Design review of the part built by this model. Coordinates are the model's own, in mm. Face numbers are marked on the shaded views. A direction names the side the tool comes from. Give positions to 0.01 mm unless a question says otherwise; leave off trailing zeros. Write each loop counter-clockwise with the first axis right and the second up, starting at its lowest first coordinate (ties: lowest second). Pieces come first, ordered by that corner, then holes.
```python
from build123d import *

# Parameters (mm, degrees)
F0_R     = 31
F1_DEPTH = 49
F2_R     = 17.5
F4_DEPTH = 52
F6_D     = 3


# Not quite as in the source:
# - the program builds the solid bodies; features that only make, move or delete a surface that nothing else refers to are left out


with BuildPart() as f1:
    # F0 (on Top) → F1 (new body)
    with BuildSketch(Plane.XY):
        Circle(F0_R)
    extrude(amount=F1_DEPTH)

    # F2 (on Top) → F4 (join)
    with BuildSketch(Plane.XY):
        Circle(F2_R)
    extrude(amount=F4_DEPTH)

    # F6 (through all)
    with Locations(Plane.XY.offset(52)):
        with Locations((0, 15), (-15, 0), (0, -15), (15, 0)):
            Hole(F6_D / 2)


solid = f1.part
```
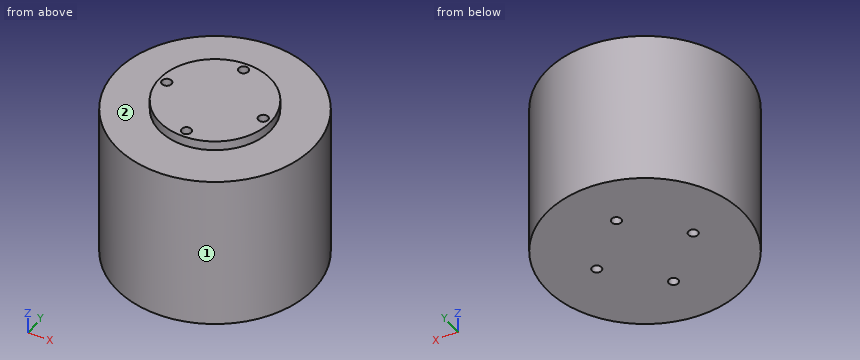
(1) Consider section D-D, the plane y = -15. Give the boundary of the cut face in (x, z).
Resolved:
outline: (-27.13, 0) - (-1.5, 0) - (-1.5, 52) - (-9.01, 52) - (-9.01, 49) - (-27.13, 49) - close; (1.5, 0) - (27.13, 0) - (27.13, 49) - (9.01, 49) - (9.01, 52) - (1.5, 52) - close
(2) Consider section A-A, the plane z = 40. Give the boundary of the cut face in (x, y), then the cut area to 3 significant figures.
Resolved:
outline: circle Ø62 at (0, 0); hole circle Ø3 at (-15, 0); hole circle Ø3 at (0, -15); hole circle Ø3 at (0, 15); hole circle Ø3 at (15, 0)
area: 2,990 mm2
(3) Clearance check with flat-ended pins moving along their axes: P1, Ø8, axis at x = 17, y = 20, coming from the +Z side; P2, Ø2, axis at y = 14.5, z = 14, coming from the -X side; P3, Ø3, axis at x = -5.5, z = 44, coming from the -Y side. State where each tip first meets the part, or that it passes through.
Resolved:
P1: stops at z = 49
P2: stops at x = -27.91
P3: stops at y = -30.74
(4) To check wall thickness, follow L1, parallel to Y at x = 0, z = 30; L2, parallel to Y at x = 1, z = 34. State the ranges of each line that lie inside material, in increasing order.
Resolved:
L1: y = -31 to -16.5, -13.5 to 13.5, 16.5 to 31
L2: y = -30.98 to -16.12, -13.88 to 13.88, 16.12 to 30.98
(5) Consider section B-B, the plane y = 0. Give the boundary of the cut face in (x, z).
Resolved:
outline: (-31, 0) - (-16.5, 0) - (-16.5, 52) - (-17.5, 52) - (-17.5, 49) - (-31, 49) - close; (-13.5, 0) - (13.5, 0) - (13.5, 52) - (-13.5, 52) - close; (16.5, 0) - (31, 0) - (31, 49) - (17.5, 49) - (17.5, 52) - (16.5, 52) - close
(6) Tool access review of the marked faces 1 and 2: name each direction out of +Z, -Z, +X, -X, +Y, -Y from which nothing blocks a thin tool from reaching the whole face with its end or side.
Resolved:
face 1: +Z, -Z
face 2: +Z
